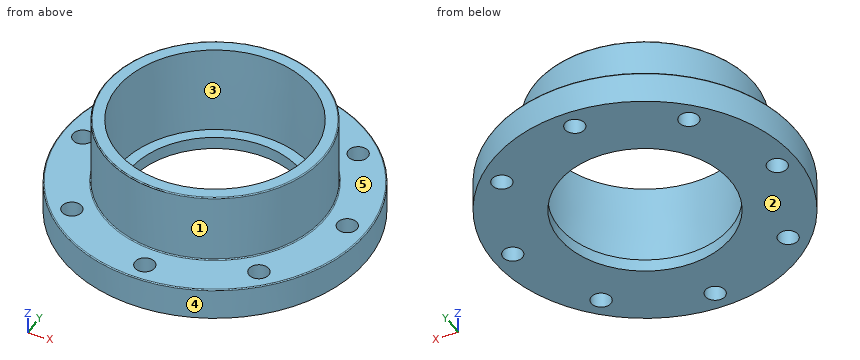
from build123d import *

# Parameters (mm, degrees)
SKETCH1_R         = 171.45
EXTRUDE1_DEPTH    = 36.5125
SKETCH2_R         = 123.825
EXTRUDE2_DEPTH    = 79.375
SKETCH3_R         = 11.1125
EXTRUDE3_DEPTH    = 256.128586452
CIRPATTERN1_COUNT = 8
FILLET1_R         = 1.154545455


with BuildPart() as part:
    # Sketch1 → Extrude1 (new body)
    with BuildSketch(Plane.XY):
        Circle(SKETCH1_R)
    extrude(amount=EXTRUDE1_DEPTH)

    # Sketch2 → Extrude2 (add)
    with BuildSketch(Plane.XY.offset(36.5125)):
        with Locations(Location((0, 0, 0), (0, 0, 180))):
            Circle(SKETCH2_R)
    extrude(amount=EXTRUDE2_DEPTH)

    # Sketch3 → Extrude3 (cut, through all)
    with BuildSketch(Plane.XY.offset(36.5125)):
        with Locations((0, 149.225)):
            Circle(SKETCH3_R)
    extrude3 = extrude(amount=-EXTRUDE3_DEPTH, mode=Mode.SUBTRACT)

    # CirPattern1: Extrude3 ×8 about axis
    cirpattern1_axis = Axis((0, 0, 0), (0, 0, 1))
    for i in range(1, CIRPATTERN1_COUNT):
        add(extrude3.rotate(cirpattern1_axis, i * 360 / CIRPATTERN1_COUNT), mode=Mode.SUBTRACT)

    # Fillet1
    fillet1_edges = [part.edges().sort_by_distance(p)[0] for p in [
        (-171.45, 0, 36.5125),
        (123.825, 0, 36.5125),
        (123.825, 0, 115.8875),
    ]]
    fillet(fillet1_edges, radius=FILLET1_R)

    # Sketch4 → Cut-Revolve1 (revolve, cut)
    with BuildSketch(Plane(origin=(0, 0, 63.5), x_dir=(0, 0, -1), z_dir=(1, 0, 0)), mode=Mode.PRIVATE) as cut_revolve1_sk:
        Polygon((-52.3875, 109.9185), (49.2125, 109.347), (49.2125, 96.8375), (63.5, 96.8375), (63.5, 0), (-52.3875, 0), align=None)
    revolve(cut_revolve1_sk.sketch.rotate(Axis((0, 0, 0), (0, 0, 1)), 270), axis=Axis((0, 0, 0), (0, 0, 1)), mode=Mode.SUBTRACT)


solid = part.part
Geometry check sheet. Reference: the model listing, model coordinates, mm. Face numbers are marked on the shaded views. A direction names the side the tool comes from. Round coordinates to 2 decimals unless told otherwise and drop trailing zeros. Write each loop counter-clockwise with the first axis right and the second up, starting at its lowest first coordinate (ties: lowest second). Pieces come first, ordered by that corner, then holes. Notation, with made-up numbers: (48.25, 57) -> (52.25, 57) arc R25 ccw to (52.25, 93) -> close; hole circle Ø5 at (28, 68.5). An arc over 180 degrees is marked (long way). One line per item, written item: value. Start each with the question number.
(1) Access from +Z, -Z, +X, -X, +Y, -Y to the whole of each face (thin tool, end or side, straight path). Record for the marked faces 4 and 5.
(2) Scan lines: line 1 (Y direction, x = 0, z = 16); line 2 (Y direction, x = 0, z = 9); line 3 (Y direction, x = 104, z = 12). Record each from-to range of solid material in increasing order. Write a range as [from, to].
(3) Cross-section at A-A, the plane y = 0. Give the number of separate pieces and of enclosed holes in the cut face, and give its area (3 significant figures).
(4) Draft check along Y on the marked faces 1, 2 and 3. Enter one of: +Y half, -Y half, draft (parallel to the pull), parting line (faces both ways), or undercut.
(5) Go/stop test with flat-tipped pins: pin 1 Ø6 at (x, z) = (-55, 94.5) entering from -Y; pin 2 Ø1.5 at (y, z) = (3, 100) entering from -X; pin 3 Ø12 at (x, z) = (-37, 43.5) entering from -Y; pin 4 Ø20 at (x, y) = (0, 149.225) entering from +Z. Record where each tip stops, or that it passes through.
(6) Cross-section at D-D, the plane z = 97. Record the cut outline in (x, y) (3 decimals).
Answer:
1. face 4: +Z, -Z
1. face 5: +Z
2. line 1: [-171.45, -160.34], [-138.11, -109.36], [109.36, 138.11], [160.34, 171.45]
2. line 2: [-171.45, -160.34], [-138.11, -96.84], [96.84, 138.11], [160.34, 171.45]
2. line 3: [-136.31, -116.53], [-94.51, 94.51], [116.53, 136.31]
3. separate pieces: 4
3. enclosed holes: 0
3. area: 5,510 mm²
4. face 1: parting line
4. face 2: draft
4. face 3: undercut
5. pin 1: y = -112.38
5. pin 2: x = -123.8
5. pin 3: y = -119.88
5. pin 4: through
6. outline: circle Ø247.65 at (0, 0); hole circle Ø219.625 at (0, 0)
